```python
from build123d import *

# Parameters (mm, degrees)
CUT_EXTRUDE1_START = -3
CUT_EXTRUDE1_DEPTH = 3
SKETCH4_R          = 2.886751346
CUT_EXTRUDE2_DEPTH = 0.5
CUT_EXTRUDE2_TAPER = 45


with BuildPart() as part:
    # Sketch2 → Revolve1 (revolve)
    with BuildSketch(Plane(origin=(0, 0, 0), x_dir=(0, 0, -1), z_dir=(1, 0, 0))):
        Polygon((-12.7, 5), (-7.3, 5), (-7, 4.7), (-7, 3), (12, 3), (13, 2), (13, 0), (-13, 0), (-13, 4.7), align=None)
    revolve(axis=Axis((0, 0, -13), (0, 0, 1)))

    # Sketch3 → Cut-Extrude1 (cut)
    with BuildSketch(Plane.XY.offset(13).offset(CUT_EXTRUDE1_START)):
        Polygon((0, 2.886751346), (-2.5, 1.443375673), (-2.5, -1.443375673), (0, -2.886751346), (2.5, -1.443375673), (2.5, 1.443375673), align=None)
    extrude(amount=CUT_EXTRUDE1_DEPTH, mode=Mode.SUBTRACT)

    # Sketch4 → Cut-Extrude2 (cut)
    with BuildSketch(Plane.XY.offset(13)):
        Circle(SKETCH4_R)
    extrude(amount=-CUT_EXTRUDE2_DEPTH, taper=CUT_EXTRUDE2_TAPER, mode=Mode.SUBTRACT)


solid = part.part
```
CAD build for the part. Positions are in the model's coordinates, mm. A direction names the side the tool comes from. Give positions to 0.01 mm unless a question says otherwise; leave off trailing zeros. Write each loop counter-clockwise with the first axis right and the second up, starting at its lowest first coordinate (ties: lowest second). Pieces come first, ordered by that corner, then holes. Notation, with made-up numbers: M -32,-39.5 L 9,-39.5 A22 ccw 9,-29.5 Z; hole C 14.5,27.25 d3. An arc over 180 degrees is marked long. Return JSON: item names as keys, results as strings. Group by question number.
(1) Band-saw the part on A-A (y = 0). Give the cut face in (x, z), and give its area (3 significant figures).
(2) Drill centre lines: L1, parallel to Z at x = 2.25, y = 2.25; L2, parallel to X at y = -0.75, z = 10.75; L3, parallel to X at y = 2, z = 10.25. Where is each one in solid material? Low to high. Write a range as [from, to].
(3) 3-axis set-ups, long thin cutter, end or side, ignore diameter. For faces 1 (the face through (1.328, -2.34, 12.804)), 2 (the face through (3, 1, 7)): which of +Z, -Z, +X, -X, +Y, -Y reach the whole face in a straight line?
(4) Mould opens along X. For faces 3 (the face through (1.233, -2.175, 11.479)), 4 (the face through (4.88, -1.08, 9.96)), 5 (the face through (0, 0, -13)) say: pulls with the +X half, pulls with the -X half, needs draft (parallel to the pull), parting line crosses it, or undercut.
(5) Band-saw the part on B-B (z = 8). Give the cut face in (x, y), and give its area (3 significant figures).
(6) Flat gauge pins, fed straight in: pin 1 Ø6 at (y, z) = (0.5, -7) entering from +X; pin 2 Ø1.5 at (x, y) = (1, -1) entering from +Z; pin 3 Ø2 at (x, z) = (2, 1) entering from +Y; pin 4 Ø3 at (x, y) = (0, 1.5) entering from +Z. Where does each tip first touch, or does it go through?
Entries:
{
 "1": {"outline": "M -5,7.3 L -4.7,7 L -3,7 L -3,-12 L -2,-13 L 2,-13 L 3,-12 L 3,7 L 4.7,7 L 5,7.3 L 5,12.7 L 4.7,13 L 2.89,13 L 2.5,12.61 L 2.5,10 L -2.5,10 L -2.5,12.61 L -2.89,13 L -4.7,13 L -5,12.7 Z", "area": "164 mm^2"},
 "2": {"L1": "z = [7, 13]", "L2": "x = [-4.94, -2.5], [2.5, 4.94]", "L3": "x = [-4.58, -1.54], [1.54, 4.58]"},
 "3": {"face 1": "+Z", "face 2": "-Z"},
 "4": {"face 3": "undercut", "face 4": "parting line crosses it", "face 5": "needs draft"},
 "5": {"outline": "C 0,0 d10", "area": "78.5 mm^2"},
 "6": {"pin 1": "stops at x = 3", "pin 2": "stops at z = 10", "pin 3": "stops at y = 2.83", "pin 4": "stops at z = 13"}
}
